Verification items for the finished model (mm, model axes). A direction names the side the tool comes from. Coordinates: 2 decimals unless noted, no trailing zeros. Order: outer loops, then holes, each group sorted by start corner. A loop starts at its lowest first (then second) coordinate and runs counter-clockwise, first axis right, second up.
Q1. Set-up check for faces 1 (the cylindrical face through (-106.913, -28.192, -24.363)), 2 (the cylindrical face through (-106.048, 28.363, -24.192)), 3 (the flat face through (2, -4.5, -14)): record each of +Z, -Z, +X, -X, +Y, -Y from which the full face is reachable in a straight line by a thin tool's end or side.
Q2. Thickness scan on line 1 (Y direction, x = 11.5, z = -12.5); line 2 (Y direction, x = -46, z = -16.5); line 3 (Z direction, x = -86, y = -13.5). Record the ranges inside material, lowest first.
Q3. Cross-section at A-A, the plane x = -73. Record the boundary of the cut face in (y, z), and give its area (3 significant figures).
Q4. Depth check by flat-ended pin: P1, Ø12, axis at x = -54.5, z = -4.5, coming from the -Y side; P2, Ø20.5, axis at x = -131.5, y = 0.5, coming from the +Z side; P3, Ø1.5, axis at y = -20, z = -6.5, coming from the +X side. Enter the tip coordinate at first touch or a pass-through.
from build123d import *

# Parameters (mm, degrees)
PAD009_DEPTH            = 60
CHAMFER_SIZE2           = 5
CHAMFER_SIZE            = 8
FILLET005_R             = 6
CHAMFER001_SIZE2        = 1.5
CHAMFER001_SIZE         = 1
PAD010_DEPTH            = 250
POCKET006_DEPTH         = 14.501
POCKET006_DEPTH_BACK    = 14.501
BODY007_ROLL_ANGLE      = -90
BODY007_PLACEMENT_ANGLE = -90


with BuildPart() as part:
    # Sketch016 → Pad009 (new body)
    with BuildSketch(Plane.XY):
        with BuildLine():
            Line((-20.5, 14.5), (20.5, 14.5))
            ThreePointArc((32.5, 2.5), (28.985281, 10.985281), (20.5, 14.5))
            Line((32.5, 2.5), (32.5, -2.5))
            ThreePointArc((20.5, -14.5), (28.985281, -10.985281), (32.5, -2.5))
            Line((20.5, -14.5), (-20.5, -14.5))
            ThreePointArc((-32.5, -2.5), (-28.985281, -10.985281), (-20.5, -14.5))
            Line((-32.5, -2.5), (-32.5, 2.5))
            ThreePointArc((-20.5, 14.5), (-28.985281, 10.985281), (-32.5, 2.5))
        make_face()
    extrude(amount=PAD009_DEPTH)

    # Chamfer
    chamfer_edges = [part.edges().sort_by_distance(p)[0] for p in [
        (0, -14.5, 60),
    ]]
    chamfer_side = part.faces().sort_by_distance((0, -14.5, 30))[0]
    chamfer(chamfer_edges, length=CHAMFER_SIZE, length2=CHAMFER_SIZE2, reference=chamfer_side)

    # Fillet005
    fillet005_edges = [part.edges().sort_by_distance(p)[0] for p in [
        (0, -14.5, 52),
        (0, -9.5, 60),
    ]]
    fillet(fillet005_edges, radius=FILLET005_R)

    # Chamfer001
    chamfer001_edges = [part.edges().sort_by_distance(p)[0] for p in [
        (28.985281, 10.985281, 0),
    ]]
    chamfer001_side = part.faces().sort_by_distance((0, 0, 0))[0]
    chamfer(chamfer001_edges, length=CHAMFER001_SIZE, length2=CHAMFER001_SIZE2, reference=chamfer001_side)

    # Chamfer001 Face10 → Pad010 (add)
    with BuildSketch(Plane(origin=(0, 0, 0), x_dir=(0, -1, 0), z_dir=(0, 0, -1))):
        with BuildLine():
            ThreePointArc((-13.5, -20.5), (-10.278175, -28.278175), (-2.5, -31.5))
            Line((-2.5, -31.5), (2.5, -31.5))
            ThreePointArc((2.5, -31.5), (10.278175, -28.278175), (13.5, -20.5))
            Line((13.5, -20.5), (13.5, 20.5))
            ThreePointArc((13.5, 20.5), (10.278175, 28.278175), (2.5, 31.5))
            Line((2.5, 31.5), (-2.5, 31.5))
            ThreePointArc((-2.5, 31.5), (-10.278175, 28.278175), (-13.5, 20.5))
            Line((-13.5, 20.5), (-13.5, -20.5))
        make_face()
    extrude(amount=PAD010_DEPTH)

    # Sketch017 → Pocket006 (cut, two sides)
    with BuildSketch(Plane.XZ) as pocket006_sk:
        with BuildLine():
            add(Edge.make_bspline(
                [(-46.924385, -167.352493), (-10.000406, -141.329865), (10.044039, -182.122086), (64.199211, -118.823822), (72.992912, -313.765839), (-68.724876, -304.271088), (-46.924385, -167.352493)],
                knots=[0, 0, 0, 0, 0.25, 0.5, 0.75, 1, 1, 1, 1], degree=3))
        make_face()
        with BuildLine():
            ThreePointArc((4.5, 40.999982), (0, 45.499982), (-4.5, 40.999982))
            Line((-4.5, 40.999982), (-4.5, 19.999982))
            ThreePointArc((-4.5, 19.999982), (0, 15.5), (4.5, 19.999982))
            Line((4.5, 19.999982), (4.5, 40.999982))
        make_face()
    extrude(amount=-POCKET006_DEPTH, mode=Mode.SUBTRACT)
    extrude(pocket006_sk.sketch, amount=POCKET006_DEPTH_BACK, mode=Mode.SUBTRACT)


with BuildPart() as part_1:
    # Body007 roll: moved
    add(part.part.rotate(Axis((0, 0, 0), (1, 0, 0)), BODY007_ROLL_ANGLE))


with BuildPart() as part_2:
    # Body007 placement: moved
    add(part_1.part.moved(Location((-28, 0, -14))).rotate(Axis((-28, 0, -14), (0, 0, 1)), BODY007_PLACEMENT_ANGLE))


solid = part_2.part
Check values:
1. face 1: -Z, -X, -Y
1. face 2: -Z, -X, +Y
1. face 3: +Z, -Z
2. line 1: y = -32.5 to -4.5, 4.5 to 32.5
2. line 2: y = -31.5 to 31.5
2. line 3: z = -27.5 to -0.5
3. outline: (-31.5, -16.5) arc R11 ccw to (-20.5, -27.5) - (20.5, -27.5) arc R11 ccw to (31.5, -16.5) - (31.5, -11.5) arc R11 ccw to (20.5, -0.5) - (-20.5, -0.5) arc R11 ccw to (-31.5, -11.5) - close
3. area: 1,600 mm2
4. P1: stops at y = -31.45
4. P2: stops at z = -0.5
4. P3: stops at x = 31.97
